```python
from build123d import *

# Parameters (mm, degrees)
F0_R     = 305
F1_DEPTH = 75
F2_T     = -3
F3_R     = 220
F4_DEPTH = 75.001


with BuildPart() as f1:
    # F0 (on Front) → F1 (new body)
    with BuildSketch(Plane.XZ):
        Circle(F0_R)
    extrude(amount=F1_DEPTH)

    # F2
    f2_openings = [f1.faces().sort_by_distance(p)[0] for p in [
        (0, 0, 0),
    ]]
    offset(amount=F2_T, openings=f2_openings)

    # F3 (on face) → F4 (cut, through all)
    with BuildSketch(Plane.XZ.offset(75)):
        Circle(F3_R)
    extrude(amount=-F4_DEPTH, mode=Mode.SUBTRACT)


solid = f1.part
```
Could you check a few things on this model? Use its own coordinates, in mm. A direction names the side the tool comes from. Round coordinates to 2 decimals unless told otherwise and drop trailing zeros. Order: outer loops, then holes, each group sorted by start corner. A loop starts at its lowest first (then second) coordinate and runs counter-clockwise, first axis right, second up. Notation, with made-up numbers: M -20,69.5 L 3,69.5 A26 cw 3,102.5 Z; hole C 51,56 d8. An arc over 180 degrees is marked long. One line per question, with ' | ' between items. Start each with the question number.
(1) Suppose I cut it at D-D on z = 228. List the corners of the cut face in (x, y) for me.
(2) Suppose I cut it at A-A on z = 0. List the corners of the cut face in (x, y) for me, then the cut area to 3 significant figures.
(3) Thinking about a two-plate mould opening in Z: for faces 1 (the face through (-47.69, -73.52, -214.77)), 2 (the face through (-295, 0, 69)), 3 (the face through (-304.705, -36.975, 13.41)), which applies, +Z half, -Z half, draft (parallel to the pull), parting line (faces both ways), or undercut?
(4) For faces 4 (the face through (21, -72, -222)), 5 (the face through (89, -75, -202)), which set-ups out of +Z, -Z, +X, -X, +Y, -Y let a thin tool reach every point of the face, with its end or its side?
(5) For P1, Ø6, axis at x = 223, z = 91.5, coming from the +Y side; P2, Ø3, axis at y = -50.5, z = -119.5, coming from the -X side; P3, Ø12, axis at x = 181.5, y = -10, coming from the +Z side, each with a flat end and sliding along its axis, tell me the tip position at first contact or that it passes through.
(6) Suppose I cut it at C-C on y = -55. List the corners of the cut face in (x, z) for me.
(7) Please list where these lines run through material, in increasing order: line 1 along Z through (x, y) = (0, -72.9); line 2 along Z through (x, y) = (7, -10.5); line 3 along X through (y, z) = (-45.5, 6).
(8) Suppose I cut it at B-B on x = 0. List the corners of the cut face in (y, z) for me, then the cut area to 3 significant figures.
Geometry results:
1) outline: M -202.59,-75 L 202.59,-75 L 202.59,0 L 198.04,0 L 198.04,-72 L -198.04,-72 L -198.04,0 L -202.59,0 Z
2) outline: M -305,-75 L -220,-75 L -220,-72 L -302,-72 L -302,0 L -305,0 Z; M 220,-75 L 305,-75 L 305,0 L 302,0 L 302,-72 L 220,-72 Z | area: 942 mm²
3) face 1: undercut | face 2: draft | face 3: parting line
4) face 4: +Y | face 5: +Z, -Z, +X, -X, -Y
5) P1: y = -72 | P2: x = -281.25 | P3: z = 249.45
6) outline: C 0,0 d610; hole C 0,0 d604
7) line 1: -305 to -220, 220 to 305 | line 2: -304.92 to -301.92, 301.92 to 304.92 | line 3: -304.94 to -301.94, 301.94 to 304.94
8) outline: M -75,-305 L 0,-305 L 0,-302 L -72,-302 L -72,-220 L -75,-220 Z; M -75,220 L -72,220 L -72,302 L 0,302 L 0,305 L -75,305 Z | area: 942 mm²
